```python
from build123d import *

# Parameters (mm, degrees)
SKETCH1_W           = 12.7
SKETCH1_H           = 63.5
BOSS_EXTRUDE1_DEPTH = 12.7
SKETCH2_W           = 10.16
SKETCH2_H           = 10.16
BOSS_EXTRUDE2_DEPTH = 10.16
SKETCH3_W           = 10.16
SKETCH3_H           = 10.16
BOSS_EXTRUDE3_DEPTH = 15.24


with BuildPart() as part:
    # Sketch1 → Boss-Extrude1 (new body)
    with BuildSketch(Plane.XY):
        with Locations((6.35, 31.75)):
            Rectangle(SKETCH1_W, SKETCH1_H)
    extrude(amount=BOSS_EXTRUDE1_DEPTH)

    # Sketch2 → Boss-Extrude2 (add)
    with BuildSketch(Plane(origin=(0, 63.5, 0), x_dir=(1, 0, 0), z_dir=(0, 1, 0))):
        with Locations((6.35, -6.35)):
            Rectangle(SKETCH2_W, SKETCH2_H)
    extrude(amount=BOSS_EXTRUDE2_DEPTH)

    # Sketch3 → Boss-Extrude3 (add)
    with BuildSketch(Plane.XZ):
        with Locations((6.35, 6.35)):
            Rectangle(SKETCH3_W, SKETCH3_H)
    extrude(amount=BOSS_EXTRUDE3_DEPTH)


solid = part.part
```
Could you check a few things on this model? Use its own coordinates, in mm. A direction names the side the tool comes from. Give positions to 0.01 mm unless a question says otherwise; leave off trailing zeros. Loops run counter-clockwise (first coordinate to the right, second up) from the corner with the lowest first, then second, coordinate; pieces in that order, holes last. Notation, with made-up numbers: (-37.75, 28.25) - (-31.75, 28.25) arc R22 cw to (-31.75, 50.25) - close; hole circle Ø4 at (45.5, 18.25). An arc over 180 degrees is marked (long way). Answer in a Markdown table with one row per item. Add a question column.
Q1. If we section it at B-B (z = 3.25): List the corners of the cut face in (x, y) for me, plus the area to 3 significant figures.
Q2. If we section it at C-C (y = -3.5): List the corners of the cut face in (x, z) for me, plus the area to 3 significant figures.
Q3. Please list where these lines run through material, in increasing order: L1, parallel to Y at x = 10.25, z = 1; L2, parallel to X at y = -8, z = 4. Write a range as from..to.
Q4. Which directions (+Z, -Z, +X, -X, +Y, -Y) give clear straight access to the entire face, cutting with the end or side of a thin tool? Please do faces 1 (the face through (6, -8, 1.27)), 2 (the face through (6, -8, 11.43)), 3 (the face through (1.27, 69, 6)), 4 (the face through (6, 69, 1.27)).
Q5. For pin 1 (1 mm diameter, centred on x = 3, y = 31.5, fed in from -Z); pin 2 (5 mm diameter, centred on y = -4, z = 8.5, fed in from -X); pin 3 (3 mm diameter, centred on x = 7.5, y = 69.5, fed in from -Z); pin 4 (3 mm diameter, centred on x = 4.5, y = -11, fed in from +Z), each with a flat end and sliding along its axis, tell me the tip position at first contact or that it passes through.
Q6. If we section it at A-A (x = 6.25): List the corners of the cut face in (y, z) for me, plus the area to 3 significant figures.
The answers:
| question | item | result |
|---|---|---|
| 1 | outline | (0, 0) - (1.27, 0) - (1.27, -15.24) - (11.43, -15.24) - (11.43, 0) - (12.7, 0) - (12.7, 63.5) - (11.43, 63.5) - (11.43, 73.66) - (1.27, 73.66) - (1.27, 63.5) - (0, 63.5) - close |
| 1 | area | 1,060 mm^2 |
| 2 | outline | (1.27, 1.27) - (11.43, 1.27) - (11.43, 11.43) - (1.27, 11.43) - close |
| 2 | area | 103 mm^2 |
| 3 | L1 | y = 0..63.5 |
| 3 | L2 | x = 1.27..11.43 |
| 4 | face 1 | -Z, +X, -X, -Y |
| 4 | face 2 | +Z, +X, -X, -Y |
| 4 | face 3 | +Z, -Z, -X, +Y |
| 4 | face 4 | -Z, +X, -X, +Y |
| 5 | pin 1 | stops at z = 0 |
| 5 | pin 2 | stops at x = 1.27 |
| 5 | pin 3 | stops at z = 1.27 |
| 5 | pin 4 | stops at z = 11.43 |
| 6 | outline | (-15.24, 1.27) - (0, 1.27) - (0, 0) - (63.5, 0) - (63.5, 1.27) - (73.66, 1.27) - (73.66, 11.43) - (63.5, 11.43) - (63.5, 12.7) - (0, 12.7) - (0, 11.43) - (-15.24, 11.43) - close |
| 6 | area | 1,060 mm^2 |
